from build123d import *

# Parameters (mm, degrees)
EXTRUDE_1_DEPTH     = 2
SKETCH_4_R          = 4.5
CUT_EXTRUDE_1_DEPTH = 98.121058479


with BuildPart() as part:
    # Эскиз2 → Бобышка-Вытянуть1 (new body)
    with BuildSketch(Plane(origin=(0, 0, 0), x_dir=(1, 0, 0), z_dir=(0, 1, 0))):
        with BuildLine():
            Line((-51.5, -58.5), (51.5, -58.5))
            ThreePointArc((51.5, -58.5), (69.884776311, -50.884776311), (77.5, -32.5))
            Line((77.5, -32.5), (77.5, 32.5))
            ThreePointArc((77.5, 32.5), (69.884776311, 50.884776311), (51.5, 58.5))
            Line((51.5, 58.5), (-51.5, 58.5))
            ThreePointArc((-51.5, 58.5), (-69.884776311, 50.884776311), (-77.5, 32.5))
            Line((-77.5, 32.5), (-77.5, -32.5))
            ThreePointArc((-77.5, -32.5), (-69.884776311, -50.884776311), (-51.5, -58.5))
        make_face()
        with BuildLine():
            Line((-51.5, 38.5), (51.5, 38.5))
            ThreePointArc((51.5, 38.5), (55.742640687, 36.742640687), (57.5, 32.5))
            Line((57.5, 32.5), (57.5, -32.5))
            ThreePointArc((57.5, -32.5), (55.742640687, -36.742640687), (51.5, -38.5))
            Line((51.5, -38.5), (-51.5, -38.5))
            ThreePointArc((-51.5, -38.5), (-55.742640687, -36.742640687), (-57.5, -32.5))
            Line((-57.5, -32.5), (-57.5, 32.5))
            ThreePointArc((-57.5, 32.5), (-55.742640687, 36.742640687), (-51.5, 38.5))
        make_face(mode=Mode.SUBTRACT)
    extrude(amount=EXTRUDE_1_DEPTH)

    # Эскиз4 → Вырез-Вытянуть1 (cut, through all)
    with BuildSketch(Plane(origin=(0, 2, 0), x_dir=(1, 0, 0), z_dir=(0, 1, 0))):
        with Locations(Location((-45, -48.5, 0), (0, 0, 270))):
            Circle(SKETCH_4_R)
    cut_extrude_1 = extrude(amount=-CUT_EXTRUDE_1_DEPTH, mode=Mode.SUBTRACT)

    # Эскиз-Массив1: Вырез-Вытянуть1 at 9 more places
    with Locations((45, 0, 0), (90, 0, 0), (112.5, 0, -23.5), (112.5, 0, -73.5), (-22.5, 0, -23.5), (-22.5, 0, -73.5), (90, 0, -97), (45, 0, -97), (0, 0, -97)):
        add(cut_extrude_1, mode=Mode.SUBTRACT)


solid = part.part
Read the model definition and answer for the solid it produces. Units are mm, in the model's axes. A direction names the side the tool comes from. Coordinates: 2 decimals unless noted, no trailing zeros. Write each loop counter-clockwise with the first axis right and the second up, starting at its lowest first coordinate (ties: lowest second). Pieces come first, ordered by that corner, then holes. Notation, with made-up numbers: (37, 82.25) -> (87, 82.25) arc R17 cw to (87, 106.25) -> close; hole circle Ø10 at (78.5, 7.25). An arc over 180 degrees is marked (long way). Return JSON: item names as keys, results as strings.
(1) For a pull along Z with two mould halves and no side action, classify faces 1 (the flat face through (-1, 0, -40)), 2 (the cylindrical face through (71.96, 1.01, -25.59)), 3 (the cylindrical face through (55.696, 0.986, -36.789)), 4 (the cylindrical face through (-69.68, 0.99, -51.09)) as pulls with the +Z half, pulls with the -Z half, needs draft (parallel to the pull), parting line crosses it, or undercut.
Answers below:
{"face 1": "needs draft", "face 2": "undercut", "face 3": "undercut", "face 4": "pulls with the -Z half"}
(2) The part is cut by section B-B on x = 0. Give the vertices of the cut face in (y, z), then the cut area to 3 significant figures.
Answers below:
{"outline": "(0, -58.5) -> (2, -58.5) -> (2, -53) -> (0, -53) -> close; (0, -44) -> (2, -44) -> (2, -38.5) -> (0, -38.5) -> close; (0, 38.5) -> (2, 38.5) -> (2, 44) -> (0, 44) -> close; (0, 53) -> (2, 53) -> (2, 58.5) -> (0, 58.5) -> close", "area": "44.0 mm^2"}
(3) Consider line 1 along X through (y, z) = (1.7, 25.5); line 2 along Z through (x, y) = (45.5, 0.15); line 3 along X through (y, z) = (0.65, -48.5). Determine where each line is inside the solid, lowest interval first. Write a range as from..to.
Answers below:
{"line 1": "-77.5..-71.97, -63.03..-57.5, 57.5..63.03, 71.97..77.5", "line 2": "-58.5..-52.97, -44.03..-38.5, 38.5..44.03, 52.97..58.5", "line 3": "-71.99..-49.5, -40.5..-4.5, 4.5..40.5, 49.5..71.99"}
(4) The part is cut by section D-D on x = 17. Give the vertices of the cut face in (y, z), then the cut area to 3 significant figures.
Answers below:
{"outline": "(0, -58.5) -> (2, -58.5) -> (2, -38.5) -> (0, -38.5) -> close; (0, 38.5) -> (2, 38.5) -> (2, 58.5) -> (0, 58.5) -> close", "area": "80.0 mm^2"}
(5) The part is cut by section C-C on y = 0.45. State how many separate pieces and enclosed holes the cut face has, then the cut area to 3 significant figures.
Answers below:
{"separate pieces": "1", "enclosed holes": "11", "area": "8,090 mm^2"}
(6) Which of the six approach directions +Z, -Z, +X, -X, +Y, -Y give full straight-line access (tool end or side, diameter ignored) to faces 5 (the cylindrical face through (-55.696, 0.986, 36.789)), 6 (the cylindrical face through (70.09, 0.99, -50.68))?
Answers below:
{"face 5": "+Y, -Y", "face 6": "-Z, +X, +Y, -Y"}
(7) This flat-tipped pin is pushed along its axis until it touches: P1, Ø14.5, axis at x = 67.5, z = 25, coming from the +Y side. Where does it stop, or does it pass through?
Answers below:
{"P1": "y = 2"}
(8) The part is cut by section A-A on z = 13.5. Give the vertices of the cut face in (x, y), then the cut area to 3 significant figures.
Answers below:
{"outline": "(-77.5, 0) -> (-57.5, 0) -> (-57.5, 2) -> (-77.5, 2) -> close; (57.5, 0) -> (77.5, 0) -> (77.5, 2) -> (57.5, 2) -> close", "area": "80.0 mm^2"}
